Build history of the part. All positions in model axes, mm. A direction names the side the tool comes from. Round coordinates to 2 decimals unless told otherwise and drop trailing zeros. Loops run counter-clockwise (first coordinate to the right, second up) from the corner with the lowest first, then second, coordinate; pieces in that order, holes last. Notation, with made-up numbers: (72, 13.25) - (81, 13.25) arc R7 ccw to (81, 18.25) - close; hole circle Ø7 at (68, 17.25). An arc over 180 degrees is marked (long way). Put each result on its own line as item: value. Start each with the question number.
from build123d import *

# Parameters (mm, degrees)
SKETCH1_W           = 180
SKETCH1_H           = 44
BOSS_EXTRUDE1_DEPTH = 1
SKETCH2_W           = 180
SKETCH2_H           = 1
BOSS_EXTRUDE2_DEPTH = 12
FILLET1_R           = 1
FILLET2_R           = 1
FILLET3_R           = 1
FILLET4_R           = 1
FILLET5_R           = 1
FILLET6_R           = 1


with BuildPart() as part:
    # Sketch1 → Boss-Extrude1 (new body)
    with BuildSketch(Plane(origin=(0, 0, 0), x_dir=(1, 0, 0), z_dir=(0, 1, 0))):
        Rectangle(SKETCH1_W, SKETCH1_H)
    extrude(amount=BOSS_EXTRUDE1_DEPTH)

    # Sketch2 → Boss-Extrude2 (add)
    with BuildSketch(Plane(origin=(0, 1, 0), x_dir=(1, 0, 0), z_dir=(0, 1, 0))):
        with Locations((0, 21.5)):
            Rectangle(SKETCH2_W, SKETCH2_H)
        with Locations((0, -21.5)):
            Rectangle(SKETCH2_W, SKETCH2_H)
    extrude(amount=BOSS_EXTRUDE2_DEPTH)

    # Fillet1
    fillet1_edges = [part.edges().sort_by_distance(p)[0] for p in [
        (0, 13, 22),
    ]]
    fillet(fillet1_edges, radius=FILLET1_R - 0.0001)  # a hair under: the kernel refuses the full size

    # Fillet2
    fillet2_edges = [part.edges().sort_by_distance(p)[0] for p in [
        (0, 13, -22),
    ]]
    fillet(fillet2_edges, radius=FILLET2_R - 0.0001)  # a hair under: the kernel refuses the full size

    # Fillet3
    fillet3_edges = [part.edges().sort_by_distance(p)[0] for p in [
        (0, 1, -21),
    ]]
    fillet(fillet3_edges, radius=FILLET3_R)

    # Fillet4
    fillet4_edges = [part.edges().sort_by_distance(p)[0] for p in [
        (0, 1, 21),
    ]]
    fillet(fillet4_edges, radius=FILLET4_R)

    # Fillet5
    fillet5_edges = [part.edges().sort_by_distance(p)[0] for p in [
        (0, 0, 22),
    ]]
    fillet(fillet5_edges, radius=FILLET5_R)

    # Fillet6
    fillet6_edges = [part.edges().sort_by_distance(p)[0] for p in [
        (0, 0, -22),
    ]]
    fillet(fillet6_edges, radius=FILLET6_R)


solid = part.part
1) Which spindle directions (+Z, -Z, +X, -X, +Y, -Y) get a long thin tool onto all of the face, cutting with end or side? Do faces 4 (the face through (-1, 1, 0)), 5 (the face through (-90, 0.7, 1.7)). Say none if no direction does.
2) Slice it at A-A, the plane y = 6.25. Write the cut outline in (x, z), and give its area (3 significant figures).
3) Drop a flat-ended pin along its axis: pin 1 Ø2 at (x, z) = (-44.5, -5) entering from +Y. Give the stop position or say it passes through.
4) Slice it at C-C, the plane z = 18.5. Write the cut outline in (x, y).
5) Pull direction Z, two halves, no side cores. Call faces 1 (the face through (-1, 7, 21)), 2 (the face through (-1, 6, 22)), 3 (the face through (90, 0.7, 1.7)): pulls with the +Z half, pulls with the -Z half, needs draft (parallel to the pull), parting line crosses it, or undercut.
6) Drill centre lines: line 1 (Z direction, x = -41, y = 4.75); line 2 (Y direction, x = -2.5, z = -3); line 3 (Y direction, x = 11, z = 20.5). Where is each one in solid material? Low to high. Write a range as [from, to].
Taken from the geometry:
1. face 4: +X, -X, +Y
1. face 5: +Z, -Z, -X, +Y, -Y
2. outline: (-90, -22) - (90, -22) - (90, -21) - (-90, -21) - close; (-90, 21) - (90, 21) - (90, 22) - (-90, 22) - close
2. area: 360 mm2
3. pin 1: stops at y = 1
4. outline: (-90, 0) - (90, 0) - (90, 1) - (-90, 1) - close
5. face 1: undercut
5. face 2: pulls with the +Z half
5. face 3: needs draft
6. line 1: z = [-22, -21], [21, 22]
6. line 2: y = [0, 1]
6. line 3: y = [0, 1.13]
